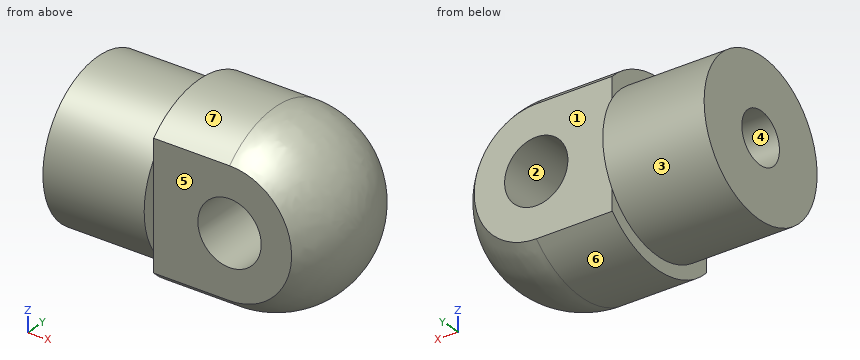
from build123d import *

# Parameters (mm, degrees)
F2_W     = 20
F2_H     = 8.8103966404
F3_DEPTH = 12.5
F4_R     = 2.5
F5_DEPTH = 25


# Not quite as in the source:
# - ends of sketch curves that miss each other by under 0.0002 mm in the source are joined


with BuildPart() as f1:
    # F0 (on Top) → F1 (revolve)
    with BuildSketch(Plane.XY):
        with BuildLine():
            Line((0, 6), (0, 2))
            Line((0, 2), (8, 2))
            Line((8, 2), (8, 0))
            Line((8, 0), (21, 0))
            ThreePointArc((21, 0), (18.9497474683, 4.9497475801), (14, 7.0000001118))
            Line((14, 7.0000001118), (8, 7.0000001118))
            Line((8, 7.0000001118), (8, 6))
            Line((8, 6), (0, 6))
        make_face()
    revolve(axis=Axis((-4.767620936, 0, 0), (-1, 0, 0)))

    # F2 (on Top) → F3 (cut, symmetric)
    with BuildSketch(Plane.XY):
        with Locations((18, -9.4051983202)):
            Rectangle(F2_W, F2_H)
        with Locations((18, 9.4051983202)):
            Rectangle(F2_W, F2_H)
    extrude(amount=F3_DEPTH, both=True, mode=Mode.SUBTRACT)

    # F4 (on face) → F5 (cut)
    with BuildSketch(Plane(origin=(0, 5, 0), x_dir=(-1, 0, 0), z_dir=(0, 1, 0))):
        with Locations((-14, 0)):
            Circle(F4_R)
    extrude(amount=-F5_DEPTH, mode=Mode.SUBTRACT)


solid = f1.part
Could you check a few things on this model? Use its own coordinates, in mm. Face numbers are marked on the shaded views. A direction names the side the tool comes from. Give positions to 0.01 mm unless a question says otherwise; leave off trailing zeros. Order: outer loops, then holes, each group sorted by start corner. A loop starts at its lowest first (then second) coordinate and runs counter-clockwise, first axis right, second up.
1. We'd pull the mould along Z, two halves only. Please class the marked faces 4, 5, 6 and 7: pulls with the +Z half, pulls with the -Z half, needs draft (parallel to the pull), parting line crosses it, or undercut.
2. Will these pins go through, and if not, where does the flat tip stop? P1, Ø6.5, axis at x = 14, z = 0, coming from the -Y side; P2, Ø1.1, axis at y = 5.5, z = 1, coming from the +X side; P3, Ø1, axis at y = 4.5, z = -2.5, coming from the -X side; P4, Ø3.5, axis at y = 0, z = 0, coming from the -X side.
3. For the marked faces 1, 2 and 3, which set-ups out of +Z, -Z, +X, -X, +Y, -Y let a thin tool reach every point of the face, with its end or its side?
4. Suppose I cut it at A-A (x = 7.75). List the corners of the cut face in (y, z) for me.
5. I need wall thicknesses on L1, parallel to Z at x = 6, y = 0; L2, parallel to Z at x = 14, y = 2.5. Which ranges of each line are inside material? Lowest first, please.
Solved:
1. face 4: undercut
1. face 5: needs draft
1. face 6: pulls with the -Z half
1. face 7: pulls with the +Z half
2. P1: stops at y = -5
2. P2: stops at x = 18.86
2. P3: stops at x = 0
2. P4: stops at x = 8
3. face 1: +Z, -Z, +X, +Y
3. face 2: +Y, -Y
3. face 3: -X
4. outline: circle Ø12 at (0, 0); hole circle Ø4 at (0, 0)
5. L1: z = -6 to -2, 2 to 6
5. L2: z = -6.54 to -2.5, 2.5 to 6.54
